Autodesk Fusion 360 part; units mm, degrees
sketch "Sketch1" plane through (0, 0, 0) normal (0, 0, 1) x (1, 0, 0)
  line L0 (0, 0) -> (70.4, 0)
  line L1 (70.4, 0) -> (70.4, -60.4)
  line L2 (70.4, -60.4) -> (0, -60.4)
  line L3 (0, -60.4) -> (0, 0)
  dimension "d1" = 60.4
  dimension "d2" = 70.4
extrude "Extrude1" add sketch "Sketch1" along normal blind 2
sketch "Sketch3" plane through (0, 0, 2) normal (0, 0, 1) x (-1, 0, 0)
  line L0 (0, 60.4) -> (-70.4, 60.4)
  line L1 (-70.4, 60.4) -> (-70.4, 0)
  line L2 (-70.4, 0) -> (0, 0)
  line L3 (0, 0) -> (0, 60.4)
  line L4 (-7.55, 25.79) -> (-65.55, 25.79)
  line L5 (-65.55, 25.79) -> (-65.55, 44.11)
  line L6 (-65.55, 44.11) -> (-7.55, 44.11)
  line L7 (-7.55, 44.11) -> (-7.55, 25.79)
  line L8 (-26, 25.79) -> (-44.32, 25.79)
  line L9 (-44.32, 25.79) -> (-44.32, 6.6)
  line L10 (-44.32, 6.6) -> (-26, 6.6)
  line L11 (-26, 6.6) -> (-26, 25.79)
  line L12 (-46.9, 60.4) -> (-8.9, 60.4)
  line L13 (-8.9, 60.4) -> (-8.9, 44.11)
  line L14 (-8.9, 44.11) -> (-46.9, 44.11)
  line L15 (-46.9, 44.11) -> (-46.9, 60.4)
  dimension "d19" = 58
  dimension "d20" = 18.32
  dimension "d21" = 7.55
  dimension "d22" = 70.4
  dimension "d23" = 18.32
  dimension "d24" = 19.19
  dimension "d25" = 6.6
  dimension "d26" = 26
  dimension "d27" = 16.29
  dimension "d28" = 38
  dimension "d29" = 8.9
extrude "Extrude2" cut sketch "Sketch3" against normal blind 2 contours L0 L6 L12 L13 L14 L15 | L4 L5 L6 L7 L8 L14 | L4 L8 L9 L10 L11
sketch "Sketch4" plane through (0, 0, 2) normal (0, 0, 1) x (-1, 0, 0)
  line L0 (-46.9, 44.11) -> (-46.9, 60.4)
  line L1 (-46.9, 60.4) -> (-70.4, 60.4)
  line L2 (-70.4, 60.4) -> (-70.4, 0)
  line L3 (-70.4, 0) -> (0, 0)
  line L4 (0, 0) -> (0, 60.4)
  line L5 (0, 60.4) -> (-8.9, 60.4)
  line L6 (-8.9, 60.4) -> (-8.9, 44.11)
  line L7 (-8.9, 44.11) -> (-7.55, 44.11)
  line L8 (-7.55, 44.11) -> (-7.55, 25.79)
  line L9 (-7.55, 25.79) -> (-26, 25.79)
  line L10 (-26, 25.79) -> (-26, 6.6)
  line L11 (-26, 6.6) -> (-44.32, 6.6)
  line L12 (-44.32, 6.6) -> (-44.32, 25.79)
  line L13 (-44.32, 25.79) -> (-65.55, 25.79)
  line L14 (-65.55, 25.79) -> (-65.55, 44.11)
  line L15 (-65.55, 44.11) -> (-46.9, 44.11)
  circle A0 centre (-56.45, 11.45) radius 8.5
  dimension "d32" = 17
  dimension "d33" = 13.95
  dimension "d34" = 11.45
extrude "Extrude3" cut sketch "Sketch4" against normal blind 2 contours A0
fillet "Fillet1" radius 1 2 edges at (8.9, -52.255, 2) (46.9, -52.255, 2)
fillet "Fillet2" radius 2 1 edges at (64.3748, -14.5237, 2)
extrude "Extrude4" add 1 faces at (55.0667, -60.4, 0.6667) along direction (0, -1, 0) blind 2
extrude "Extrude5" add 1 faces at (5.6, -60.4, 0.6667) along direction (0, -1, 0) blind 2
extrude "Extrude6" add 1 faces at (0, -41.6, 1.3333) along direction (-1, 0, 0) blind 2
extrude "Extrude7" add 1 faces at (46.2667, 0, 0.6667) along direction (0, 1, 0) blind 2
extrude "Extrude13" add 1 faces at (70.4, -40.9333, 0.6667) along direction (1, 0, 0) blind 2
extrude "Extrude14" add 2 faces at (4.9333, -62.4, 0.6667) (55.7333, -62.4, 0.6667) along direction (0, -1, 0) blind 2.1
extrude "Extrude15" add 1 faces at (72.4, -42.3333, 0.6667) along direction (1, 0, 0) blind 2.1
extrude "Extrude16" add 1 faces at (49, 2, 1.3333) along direction (0, 1, 0) blind 2.1
extrude "Extrude17" add 1 faces at (-2, -18.7667, 1.3333) along direction (-1, 0, 0) blind 2.1
sketch "Sketch6" plane through (0, 0, 0) normal (0, 0, -1) x (1, 0, 0)
  circle A0 centre (56.45, 11.45) radius 8.5
  line L0 (46.9, 64.5) -> (46.9, 44.11)
  line L1 (46.9, 44.11) -> (65.55, 44.11)
  line L2 (65.55, 44.11) -> (65.55, 25.79)
  line L3 (65.55, 25.79) -> (44.32, 25.79)
  line L4 (44.32, 25.79) -> (44.32, 6.6)
  line L5 (44.32, 6.6) -> (26, 6.6)
  line L6 (26, 6.6) -> (26, 25.79)
  line L7 (26, 25.79) -> (7.55, 25.79)
  line L8 (7.55, 25.79) -> (7.55, 44.11)
  line L9 (7.55, 44.11) -> (8.9, 44.11)
  line L10 (8.9, 44.11) -> (8.9, 64.5)
  line L11 (8.9, 64.5) -> (-4.1, 64.5)
  line L12 (-4.1, 64.5) -> (-4.1, -4.1)
  line L13 (-4.1, -4.1) -> (74.5, -4.1)
  line L14 (74.5, -4.1) -> (74.5, 64.5)
  line L15 (74.5, 64.5) -> (46.9, 64.5)
  line L16 (-4.1, -4.1) -> (74.5, -4.1)
  line L17 (74.5, -4.1) -> (74.5, -2.1)
  line L18 (74.5, -2.1) -> (-4.1, -2.1)
  line L19 (-4.1, -2.1) -> (-4.1, -4.1)
  line L20 (74.5, -4.1) -> (72.5, -4.1)
  line L21 (72.5, -4.1) -> (72.5, 64.5)
  line L22 (72.5, 64.5) -> (74.5, 64.5)
  line L23 (74.5, 64.5) -> (74.5, -4.1)
  line L24 (-4.1, 64.5) -> (-2.1, 64.5)
  line L25 (-2.1, 64.5) -> (-2.1, -4.1)
  line L26 (-2.1, -4.1) -> (-4.1, -4.1)
  line L27 (-4.1, -4.1) -> (-4.1, 64.5)
  line L28 (-4.1, 64.5) -> (8.9, 64.5)
  line L29 (8.9, 64.5) -> (8.9, 62.5)
  line L30 (8.9, 62.5) -> (-4.1, 62.5)
  line L31 (-4.1, 62.5) -> (-4.1, 64.5)
  line L32 (46.9, 64.5) -> (74.5, 64.5)
  line L33 (74.5, 64.5) -> (74.5, 62.5)
  line L34 (74.5, 62.5) -> (46.9, 62.5)
  line L35 (46.9, 62.5) -> (46.9, 64.5)
  dimension "d69" = 2
  dimension "d70" = 2
  dimension "d71" = 2
  dimension "d72" = 2
  dimension "d73" = 2
extrude "Extrude18" add sketch "Sketch6" along normal blind 4 contours L0 L15 L21 L32 L34 L35 | L14 L15 L21 L22 L23 L32 L33 L34 | L14 L18 L21 L23 L34 | L13 L16 L18 L21 L25 | L13 L14 L16 L17 L18 L20 L21 L23 | L12 L13 L16 L18 L19 L25 L26 L27 | L12 L18 L25 L27 L30 | L11 L12 L24 L25 L27 L28 L30 L31 | L10 L11 L25 L28 L29 L30
sketch "Sketch7" plane through (8.9, 0, 0) normal (1, 0, 0) x (0, 1, 0)
  line L0 (-44.11, 1) -> (-64.5, 1)
  line L1 (-64.5, 1) -> (-64.5, -4)
  line L2 (-64.5, -4) -> (-62.5, -4)
  line L3 (-62.5, -4) -> (-62.5, 0)
  line L4 (-62.5, 0) -> (-44.11, 0)
  line L5 (-44.11, 0) -> (-44.11, 1)
  line L6 (-62.5, -4) -> (-64.5, -4)
  line L7 (-64.5, -4) -> (-64.5, 1)
  line L8 (-64.5, 1) -> (-62.5, 1)
  line L9 (-62.5, 1) -> (-62.5, -4)
extrude "Extrude19" add sketch "Sketch7" along normal blind 38 contours L0 L1 L2 L3 L6 L7 L8 L9
Part model, mm, in its own coordinate system. A direction names the side the tool comes from. Coordinates: 2 decimals unless noted, no trailing zeros. Loops run counter-clockwise (first coordinate to the right, second up) from the corner with the lowest first, then second, coordinate; pieces in that order, holes last. Notation, with made-up numbers: M 76.25,77 L 134.25,77 A36 ccw 134.25,111 Z; hole C -20.75,40.5 d8. An arc over 180 degrees is marked long. Use a Markdown table: item, result. Add a question column.
Q1. Cut at D-D (x = 29). Write the cut outline in (y, z).
Q2. Cut at A-A (y = -11.45). Give the number of separate pieces and of enclosed holes in the cut face, and give its area (3 significant figures).
Q3. Pin check, flat tips, straight feed: P1, Ø2, axis at x = 12, y = -23.5, coming from the -Z side; P2, Ø13.5, axis at x = 56.45, y = -11.45, coming from the -Z side; P3, Ø2, axis at x = 36.5, y = -63.5, coming from the +Z side. Stop position of each tip, or through.
Q4. Cut at C-C (y = -32). Write the cut outline in (x, z).
Q5. Which spindle directions (+Z, -Z, +X, -X, +Y, -Y) get a long thin tool onto all of the face, cutting with end or side? Do faces 1 (the flat face through (44.32, -16, 1)), 2 (the flat face through (28, -63, 1)), 3 (the flat face through (36, 2.1, -2)), 4 (the flat face through (-4.1, -31, -1)). Say none if no direction does.
Q6. Mould opens along Y. For faces 5 (the flat face through (36, 4.1, -1)), 6 (the flat face through (72.5, -30, -2)), 7 (the flat face through (35, -64.5, -1)), 8 (the flat face through (56, -44.11, 1)) say: +Y half, -Y half, draft (parallel to the pull), parting line (faces both ways), or undercut.
Q7. Probe L1, parallel to Y at x = 56.45, z = 0.05; L2, parallel to Y at x = 30, z = -0.45; L3, parallel to Y at x = 46, z = 0.15. List the from-to ranges inside material, lowest first.
Worked out:
| question | item | result |
|---|---|---|
| 1 | outline | M -64.5,-4 L -62.5,-4 L -62.5,1 L -64.5,1 Z; M -6.6,0 L 2.1,0 L 2.1,-4 L 4.1,-4 L 4.1,2 L -6.6,2 Z |
| 2 | separate pieces | 3 |
| 2 | enclosed holes | 0 |
| 2 | area | 101 mm2 |
| 3 | P1 | stops at z = 0 |
| 3 | P2 | passes through |
| 3 | P3 | stops at z = 1 |
| 4 | outline | M -4.1,-4 L -2.1,-4 L -2.1,0 L 7.55,0 L 7.55,2 L -4.1,2 Z; M 65.55,0 L 72.5,0 L 72.5,-4 L 74.5,-4 L 74.5,2 L 65.55,2 Z |
| 5 | face 1 | +Z, -Z |
| 5 | face 2 | +Z, -Y |
| 5 | face 3 | -Z |
| 5 | face 4 | +Z, -Z, -X, +Y, -Y |
| 6 | face 5 | +Y half |
| 6 | face 6 | undercut |
| 6 | face 7 | -Y half |
| 6 | face 8 | undercut |
| 7 | L1 | y = -64.5 to -44.11, -25.79 to -19.95, -2.95 to 4.1 |
| 7 | L2 | y = -64.5 to -62.5, 2.1 to 4.1 |
| 7 | L3 | y = -64.5 to -62.5, -25.79 to 4.1 |
